For this review, use the dimensioned drawing (mm, ordinates from the lowest corner) and the shaded views. Round coordinates to 2 decimals unless told otherwise and drop trailing zeros. Write each loop counter-clockwise with the first axis right and the second up, starting at its lowest first coordinate (ties: lowest second). Pieces come first, ordered by that corner, then holes.
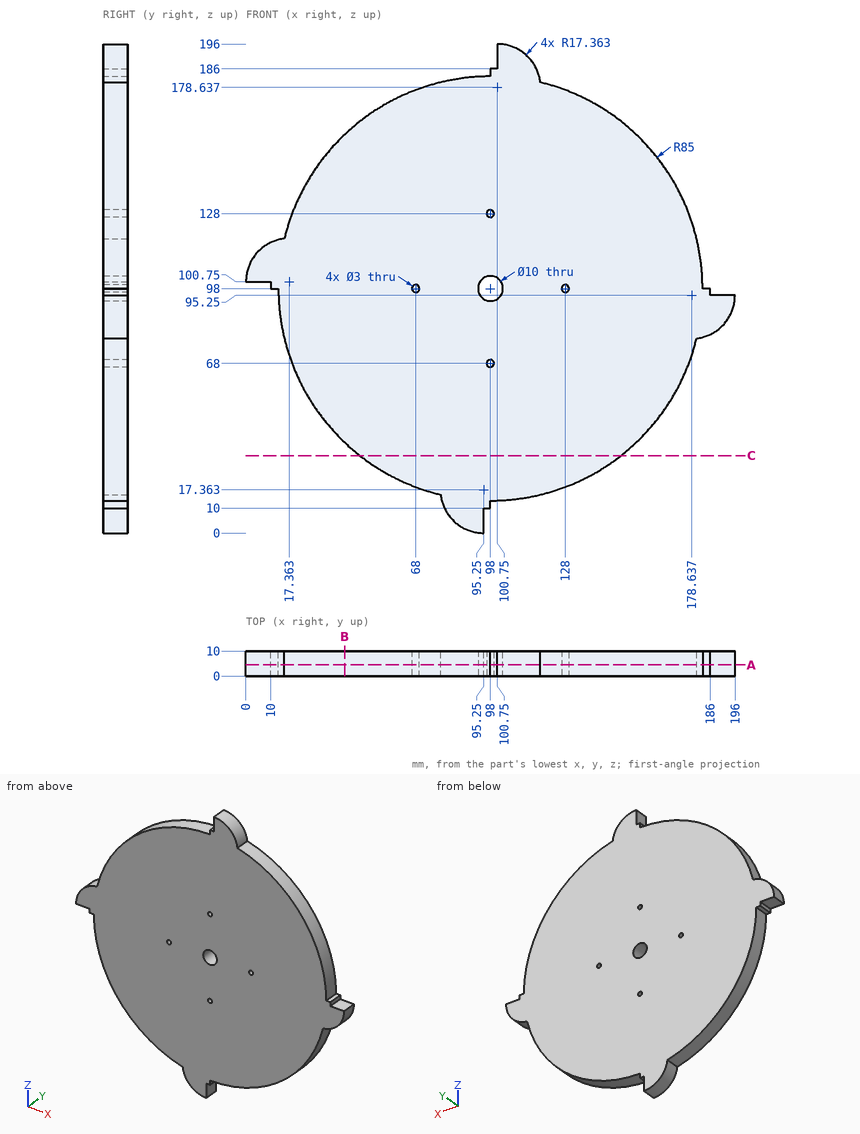
(1) For pin 1 Ø1.4 at (x, y) = (97, 6.5) entering from -Z; pin 2 Ø3 at (x, y) = (4.5, 6.5) entering from -Z; pin 3 Ø2.5 at (x, z) = (98, 68) entering from +Y (3 decimals); pin 4 Ø2.5 at (y, z) = (4, 185) entering from -X, all flat-tipped, find the tip position at first contact; note any pin that passes through.
Geometry check:
pin 1: stops at z = 10
pin 2: stops at z = 100.75
pin 3: passes through
pin 4: stops at x = 98
(2) We need section B-B, the plane x = 39.5. Give the boundary of the cut face in (y, z).
Geometry check:
outline: (0, 36.33) - (10, 36.33) - (10, 159.67) - (0, 159.67) - close
(3) For line 1 along Z through (x, y) = (128, 7); line 2 along X through (y, z) = (1.5, 102.5); line 3 along Z through (x, y) = (87, 8) (1 decimal), list the stretches that pass through material, from the lowest coordinate up.
Geometry check:
line 1: z = 18.47 to 96.5, 99.5 to 177.53
line 2: x = 0.09 to 95.82, 100.18 to 182.88
line 3: z = 2.1 to 182.3
(4) We need section C-C, the plane z = 31. Give the boundary of the cut face in (x, y).
Geometry check:
outline: (45.69, 0) - (150.31, 0) - (150.31, 10) - (45.69, 10) - close
(5) We need section A-A, the plane y = 4.5. Give the boundary of the cut face in (x, z).
Geometry check:
outline: (0, 100.75) - (10, 100.75) - (10, 98) - (13, 98) arc R85 ccw to (78, 15.39) arc R17.36 ccw to (95.25, 0) - (95.25, 10) - (98, 10) - (98, 13) arc R85 ccw to (180.61, 78) arc R17.36 ccw to (196, 95.25) - (186, 95.25) - (186, 98) - (183, 98) arc R85 ccw to (118, 180.61) arc R17.36 ccw to (100.75, 196) - (100.75, 186) - (98, 186) - (98, 183) arc R85 ccw to (15.39, 118) arc R17.36 ccw to start; hole circle Ø3 at (68, 98); hole circle Ø10 at (98, 98); hole circle Ø3 at (98, 68); hole circle Ø3 at (98, 128); hole circle Ø3 at (128, 98)
